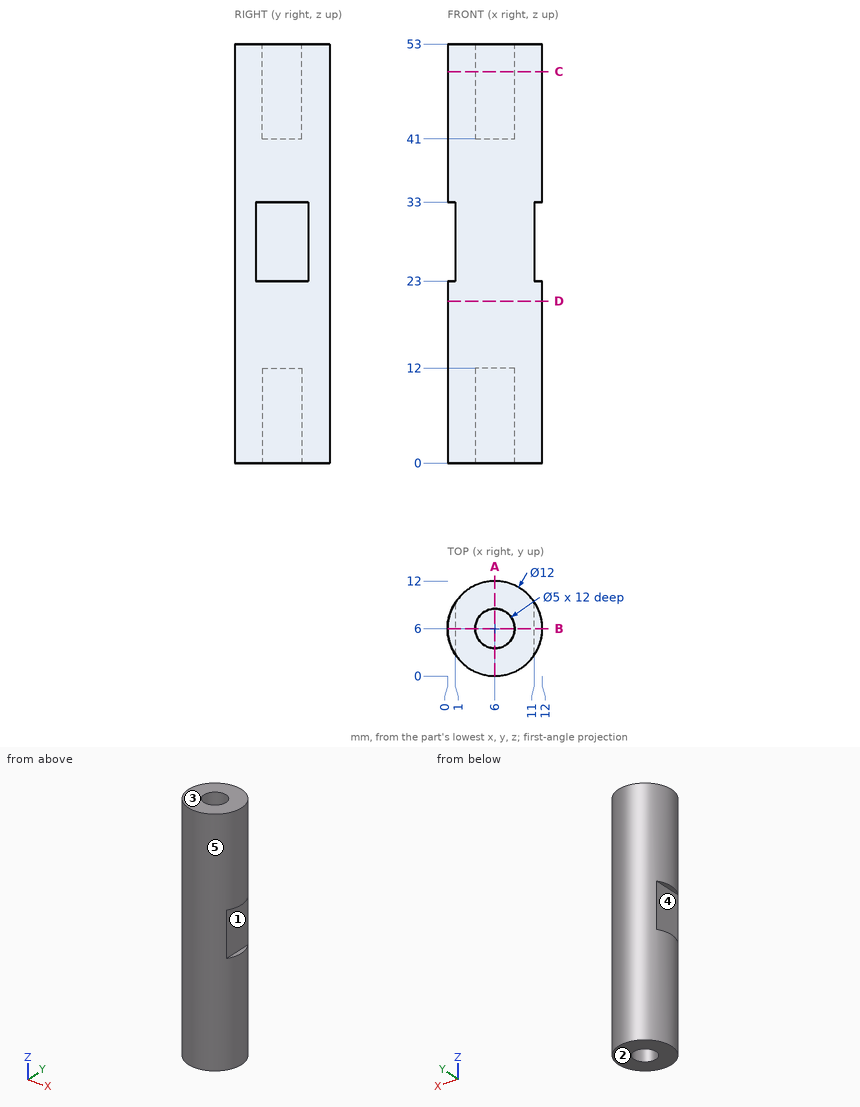
Drawing for the job (mm, zero at the part's lowest x, y, z). A direction names the side the tool comes from. Round coordinates to 2 decimals unless told otherwise and drop trailing zeros. Loops run counter-clockwise (first coordinate to the right, second up) from the corner with the lowest first, then second, coordinate; pieces in that order, holes last. Notation, with made-up numbers: (62.5, -16) -> (115.5, -16) arc R19 cw to (115.5, -7) -> close; hole circle Ø9 at (3.25, 35). An arc over 180 degrees is marked (long way). Use one line per item in the form item = value. Start each with the question number.
Item 1: Band-saw the part on B-B (y = 6). List the corners of the cut face in (x, z).
Item 2: Band-saw the part on C-C (z = 49.5). List the corners of the cut face in (x, y), plus the area to 3 significant figures.
Item 3: Drop flat-ended pins along their axis: pin 1 Ø1.5 at (x, y) = (5, 6.5) entering from -Z; pin 2 Ø6 at (y, z) = (2.5, 24.5) entering from -X; pin 3 Ø1.5 at (x, z) = (8, 23) entering from -Y. Give the stop position or say it passes through.
Item 4: Drill centre lines: line 1 along X through (y, z) = (6, 49); line 2 along X through (y, z) = (4, 7.5). Where is each one in solid material? Low to high.
Item 5: Band-saw the part on D-D (z = 20.5). List the corners of the cut face in (x, y), plus the area to 3 significant figures.
Item 6: Tool access for the marked faces 4 and 5: list every direction of +Z, -Z, +X, -X, +Y, -Y with a clear straight run to the whole face (end or side of a thin tool).
Item 7: Two-plate mould, pull along Z, no slides. Class the marked faces 1, 2 and 3: released by +Z, released by -Z, zero draft, split by the parting line, or undercut.
Item 8: Band-saw the part on A-A (x = 6). List the corners of the cut face in (y, z), plus the area to 3 significant figures.
Data:
q1.outline = (0, 0) -> (3.5, 0) -> (3.5, 12) -> (8.5, 12) -> (8.5, 0) -> (12, 0) -> (12, 23) -> (11, 23) -> (11, 33) -> (12, 33) -> (12, 53) -> (8.5, 53) -> (8.5, 41) -> (3.5, 41) -> (3.5, 53) -> (0, 53) -> (0, 33) -> (1, 33) -> (1, 23) -> (0, 23) -> close
q2.outline = circle Ø12 at (6, 6); hole circle Ø5 at (6, 6)
q2.area = 93.5 mm^2
q3.pin_1 = 12
q3.pin_2 = 0.07
q3.pin_3 = 0.13
q4.line_1 = 0 to 3.5, 8.5 to 12
q4.line_2 = 0.34 to 4.5, 7.5 to 11.66
q5.outline = circle Ø12 at (6, 6)
q5.area = 113 mm^2
q6.face_4 = -X, +Y, -Y
q6.face_5 = +Z, -Z
q7.face_1 = undercut
q7.face_2 = released by -Z
q7.face_3 = released by +Z
q8.outline = (0, 0) -> (3.5, 0) -> (3.5, 12) -> (8.5, 12) -> (8.5, 0) -> (12, 0) -> (12, 53) -> (8.5, 53) -> (8.5, 41) -> (3.5, 41) -> (3.5, 53) -> (0, 53) -> close
q8.area = 516 mm^2
